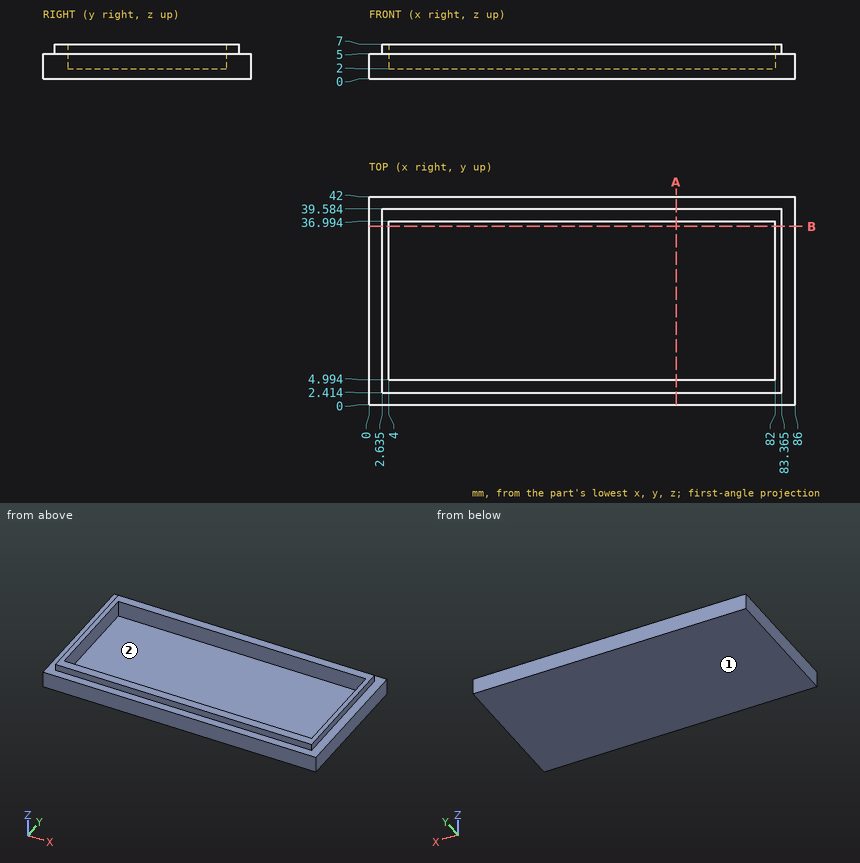
Check sheet for the drawn part. Datum: minimum x, y, z corner. Units: mm. Round coordinates to 2 decimals unless told otherwise and drop trailing zeros. Loops run counter-clockwise (first coordinate to the right, second up) from the corner with the lowest first, then second, coordinate; pieces in that order, holes last. Notation, with made-up numbers: M -24.75,51.25 L 25.25,51.25 A18 cw 25.25,73.25 Z; hole C 87,82.5 d4. An arc over 180 degrees is marked long. Write each question's results on one line, items separated by ' | '.
1) Section check B-B on y = 36. Record the boundary of the cut face in (x, z) (1 decimal).
Checks:
outline: M 0,0 L 86,0 L 86,5 L 83.4,5 L 83.4,7 L 82,7 L 82,2 L 4,2 L 4,7 L 2.6,7 L 2.6,5 L 0,5 Z
2) Scan lines: L1, parallel to Y at x = 16, z = 4; L2, parallel to X at y = 6.5, z = 4.5; L3, parallel to X at y = 15.5, z = 6 (1 decimal). Record each from-to range of solid material in increasing order. Write a range as from..to.
Checks:
L1: y = 0..4.99, 36.99..42 | L2: x = 0..4, 82..86 | L3: x = 2.6..4, 82..83.4
3) Mould release check, pull along X, two halves, no side actions. Record for the marked faces 1 and 2: released by +X, released by -X, zero draft, split by the parting line, or undercut.
Checks:
face 1: zero draft | face 2: undercut
4) Gauge pin test, flat ends, axial feed: P1, Ø0.6, axis at x = 29.5, z = 5.5, coming from the +Y side (1 decimal); P2, Ø16, axis at x = 57.5, y = 17, coming from the +Z side; P3, Ø0.6, axis at y = 12.5, z = 6.5, coming from the -X side (1 decimal). Record the tip position at first contact, or that the pin passes through.
Checks:
P1: stops at y = 39.6 | P2: stops at z = 2 | P3: stops at x = 2.6
5) Section check A-A on x = 62. Record the boundary of the cut face in (y, z) (1 decimal), then the cut area to 3 significant figures.
Checks:
outline: M 0,0 L 42,0 L 42,5 L 39.6,5 L 39.6,7 L 37,7 L 37,2 L 5,2 L 5,7 L 2.4,7 L 2.4,5 L 0,5 Z | area: 124 mm2
